Source: CAD feature listing. Evaluate the final solid. Frame: model axes, mm. A direction names the side the tool comes from. Round coordinates to 2 decimals unless told otherwise and drop trailing zeros. Order: outer loops, then holes, each group sorted by start corner. A loop starts at its lowest first (then second) coordinate and runs counter-clockwise, first axis right, second up. Notation, with made-up numbers: (83.5, -1.75) -> (102.5, -1.75) arc R23 cw to (102.5, 37.25) -> close; hole circle Ø7 at (-22.75, 80.5). An arc over 180 degrees is marked (long way). Use a Markdown table: item, result. Add a question column.
```python
from build123d import *

# Parameters (mm, degrees)
BASPROSKE_W         = 6
BASPROSKE_H         = 11.25
TOOTHCUT_DEPTH      = 18.003676073
TEETHCUTS_COUNT     = 16
TEETHCUTS_ANGLE     = 337.5
BORSKE_R            = 3
BORE_DEPTH          = 50.0000508
SKETCH_1_W          = 7.5
SKETCH_1_H          = 12
CUT_EXTRUDE_1_DEPTH = 2


with BuildPart() as part:
    # BasProSke → Base-Revolve (revolve)
    with BuildSketch(Plane(origin=(0, 0, 0), x_dir=(1, 0, 0), z_dir=(0, 1, 0)), mode=Mode.PRIVATE) as base_revolve_sk:
        with Locations((3, 5.625)):
            Rectangle(BASPROSKE_W, BASPROSKE_H)
    revolve(base_revolve_sk.sketch.rotate(Axis((-10, 0, 0), (1, 0, 0)), 180), axis=Axis((-10, 0, 0), (1, 0, 0)))

    # TooCutSke → ToothCut (cut, through all)
    with BuildSketch(Plane(origin=(0, 0, 0), x_dir=(0, 0, -1), z_dir=(1, 0, 0))):
        with BuildLine():
            ThreePointArc((0.651061533, 8.411340626), (0, 8.4365), (-0.651061533, 8.411340626))
            ThreePointArc((-0.651061533, 8.411340626), (-1.029874156, 9.883978829), (-1.930926138, 11.108832945))
            ThreePointArc((-1.930926138, 11.108832945), (0, 11.2754), (1.930926138, 11.108832945))
            ThreePointArc((1.930926138, 11.108832945), (1.029874156, 9.883978829), (0.651061533, 8.411340626))
        make_face()
    toothcut = extrude(amount=TOOTHCUT_DEPTH, mode=Mode.SUBTRACT)

    # TeethCuts: ToothCut ×16 about axis
    teethcuts_axis = Axis((-10, 0, 0), (1, 0, 0))
    for i in range(1, TEETHCUTS_COUNT):
        add(toothcut.rotate(teethcuts_axis, i * TEETHCUTS_ANGLE / (TEETHCUTS_COUNT - 1)), mode=Mode.SUBTRACT)

    # BorSke → Bore (cut, symmetric)
    with BuildSketch(Plane(origin=(0, 0, 0), x_dir=(0, 0, -1), z_dir=(1, 0, 0))):
        with Locations(Location((0, 0, 0), (0, 0, 180))):
            Circle(BORSKE_R)
    extrude(amount=BORE_DEPTH, both=True, mode=Mode.SUBTRACT)

    # Эскиз1 → Вырез-Вытянуть1 (cut)
    with BuildSketch(Plane(origin=(6, 0, 0), x_dir=(0, 0, -1), z_dir=(1, 0, 0))):
        Rectangle(SKETCH_1_W, SKETCH_1_H)
    extrude(amount=-CUT_EXTRUDE_1_DEPTH, mode=Mode.SUBTRACT)


solid = part.part
```
1) Section C-C on y = -4.5. Output: boundary loops of the cut face in (x, z), then the cut area to 3 significant figures.
2) Section D-D on y = -6.75. Output: boundary loops of the cut face in (x, z), then the cut area to 3 significant figures.
3) Section A-A on y = 0. Output: boundary loops of the cut face in (x, z).
4) Reachability of faces 1 (the flat face through (5, 0, -3.75)), 2 (the cylindrical face through (2.96, -5.97, -5.96)), 3 (the cylindrical face through (2.958, 8.712, 4.706)) from +Z, -Z, +X, -X, +Y, -Y: full face, straight path, thin tool, end or side. Return the list, or none.
5) Section B-B on z = 0. Output: boundary loops of the cut face in (x, y).
6) Line query: probe 1 along Z at (x, y) = (3.1, 9.25); probe 2 along Z at (x, y) = (1.45, -6); probe 3 along Z at (x, y) = (1.05, -9). Output: solid intervals per line, ascending. Write a range as from..to.
7) First-contact query: pin 1 Ø1 at (y, z) = (3, -2) entering from +X; pin 2 Ø5.5 at (y, z) = (0, 0) entering from +X; pin 3 Ø0.6 at (x, y) = (4.5, 1) entering from -Z; pin 4 Ø0.6 at (x, y) = (5, -1) entering from +Z. Flat tips, straight axial feed; report the tip coordinate or a pass-through.
Conclusion:
| question | item | result |
|---|---|---|
| 1 | outline | (0, -8.51) -> (6, -8.51) -> (6, -3.75) -> (4, -3.75) -> (4, 3.75) -> (6, 3.75) -> (6, 8.51) -> (0, 8.51) -> close |
| 1 | area | 87.1 mm^2 |
| 2 | outline | (0, -5.76) -> (6, -5.76) -> (6, 5.76) -> (0, 5.76) -> close |
| 2 | area | 69.1 mm^2 |
| 3 | outline | (0, -8.44) -> (6, -8.44) -> (6, -3.75) -> (4, -3.75) -> (4, -3) -> (0, -3) -> close; (0, 3) -> (4, 3) -> (4, 3.75) -> (6, 3.75) -> (6, 8.44) -> (0, 8.44) -> close |
| 4 | face 1 | +X |
| 4 | face 2 | +X, -X |
| 4 | face 3 | +X, -X, +Y |
| 5 | outline | (0, -8.44) -> (6, -8.44) -> (6, -6) -> (4, -6) -> (4, -3) -> (0, -3) -> close; (0, 3) -> (4, 3) -> (4, 6) -> (6, 6) -> (6, 8.44) -> (0, 8.44) -> close |
| 6 | probe 1 | z = -6.4..-5.44, -2.84..-0.79, 0.79..2.84, 5.44..6.4 |
| 6 | probe 2 | z = -9.51..-7.14, -5.93..5.93, 7.14..9.51 |
| 6 | probe 3 | z = -6.49..-5.06, -2.82..-0.73, 0.73..2.82, 5.06..6.49 |
| 7 | pin 1 | stops at x = 4 |
| 7 | pin 2 | passes through |
| 7 | pin 3 | stops at z = -10.36 |
| 7 | pin 4 | stops at z = 10.36 |
